Can you work these out from the model? Positions are in its coordinate system, mm. A direction names the side the tool comes from. Coordinates: 2 decimals unless noted, no trailing zeros. Order: outer loops, then holes, each group sorted by start corner. A loop starts at its lowest first (then second) coordinate and runs counter-clockwise, first axis right, second up. Notation, with made-up numbers: (-34, 3.5) - (-3, 3.5) arc R16 cw to (-3, 10.5) - close; hole circle Ø11 at (16, -19.75). An arc over 180 degrees is marked (long way). Return JSON: item names as keys, results as strings. Group by question number.
1) Which directions (+Z, -Z, +X, -X, +Y, -Y) give clear straight access to the entire face, cutting with the end or side of a thin tool? Please do faces 5 (the face through (32, -2, 0)), 6 (the face through (62, -2.5, 43)).
2) If we mould it in two halves opening along X, with no side actions, what happens to faces 1 (the face through (65, -2, 22)), 2 (the face through (2.34, -3.73, 43.74)), 3 (the face through (0, -2, 22)), 4 (the face through (63.69, -3.73, 2.88))? For each: pulls with the +X half, pulls with the -X half, needs draft (parallel to the pull), parting line crosses it, or undercut.
3) For pin 1 Ø1.2 at (x, z) = (62.5, 42.5) entering from -Y, with a flat end and sliding along its axis, tell me the tip position at first contact or that it passes through.
4) Imagine slicing it at A-A (z = 2.5). Write out the boundary of the cut face in (x, y), and give its area (4 significant figures).
5) Imagine slicing it at B-B (x = 62.5). Write out the boundary of the cut face in (y, z), and give its area (4 significant figures).
6) If I drill on line 1 along Z through (x, y) = (62.5, -4.3), over which ranges is the centre line in solid material (lowest first)?
```python
from build123d import *

# Parameters (mm, degrees)
F0_W     = 65
F0_H     = 45
F0_R     = 1.25
F1_DEPTH = 5
F2_DEPTH = 2.5


with BuildPart() as f1:
    # F0 (on Front) → F1 (new body)
    with BuildSketch(Plane.XZ):
        with Locations((32.5, 22.5)):
            Rectangle(F0_W, F0_H)
        with Locations((2.5, 2.5)):
            Circle(F0_R, mode=Mode.SUBTRACT)
        with Locations((62.5, 2.5)):
            Circle(F0_R, mode=Mode.SUBTRACT)
        with Locations((2.5, 42.5)):
            Circle(F0_R, mode=Mode.SUBTRACT)
        with Locations((62.5, 42.5)):
            Circle(F0_R, mode=Mode.SUBTRACT)
    extrude(amount=F1_DEPTH)

    # F0 (on Front) → F2 (join)
    with BuildSketch(Plane.XZ):
        with Locations((2.5, 42.5)):
            Circle(F0_R)
        with Locations((2.5, 2.5)):
            Circle(F0_R)
        with Locations((62.5, 2.5)):
            Circle(F0_R)
        with Locations((62.5, 42.5)):
            Circle(F0_R)
    extrude(amount=F2_DEPTH)


solid = f1.part
```
Calculated:
{
 "1": {"face 5": "-Z, +X, -X, +Y, -Y", "face 6": "-Y"},
 "2": {"face 1": "pulls with the +X half", "face 2": "undercut", "face 3": "pulls with the -X half", "face 4": "undercut"},
 "3": {"pin 1": "y = -2.5"},
 "4": {"outline": "(0, -5) - (1.25, -5) - (1.25, -2.5) - (3.75, -2.5) - (3.75, -5) - (61.25, -5) - (61.25, -2.5) - (63.75, -2.5) - (63.75, -5) - (65, -5) - (65, 0) - (0, 0) - close", "area": "312.5 mm2"},
 "5": {"outline": "(-5, 0) - (0, 0) - (0, 45) - (-5, 45) - (-5, 43.75) - (-2.5, 43.75) - (-2.5, 41.25) - (-5, 41.25) - (-5, 3.75) - (-2.5, 3.75) - (-2.5, 1.25) - (-5, 1.25) - close", "area": "212.5 mm2"},
 "6": {"line 1": "0 to 1.25, 3.75 to 41.25, 43.75 to 45"}
}
